Read the model definition and answer for the solid it produces. Units are mm, in the model's axes. Coordinates: 2 decimals unless noted, no trailing zeros. Write each loop counter-clockwise with the first axis right and the second up, starting at its lowest first coordinate (ties: lowest second). Pieces come first, ordered by that corner, then holes. Notation, with made-up numbers: (39, -9) -> (54, -9) arc R36 ccw to (54, 28) -> close; hole circle Ø4 at (-11, 56.5). An arc over 180 degrees is marked (long way). Use CSV: the item, a comma, the result in double quotes.
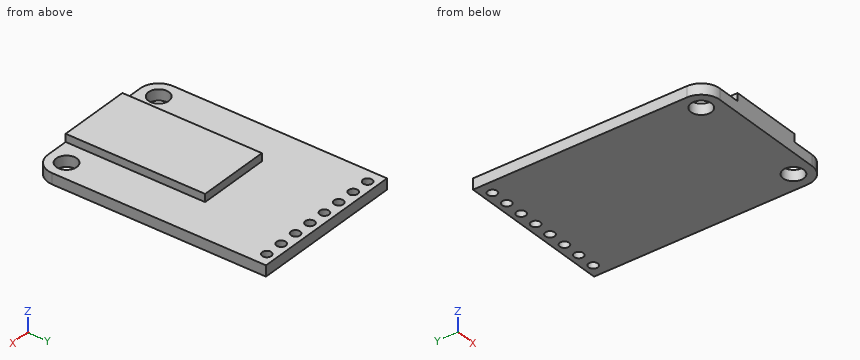
from build123d import *

# Parameters (mm, degrees)
F0_W     = 21.336
F0_H     = 31.75
F1_DEPTH = 1.4732
F2_R     = 2.54
F3_R     = 1.397
F4_DEPTH = 1.4732
F5_R     = 0.635
F6_DEPTH = 1.4732
F7_W     = 10.0076
F7_H     = 19.05
F8_DEPTH = 2.54


with BuildPart() as f1:
    # F0 (on Top) → F1 (new body)
    with BuildSketch(Plane.XY):
        Rectangle(F0_W, F0_H)
    extrude(amount=F1_DEPTH)

    # F2
    f2_edges = [f1.edges().sort_by_distance(p)[0] for p in [
        (10.668, -15.875, 0.7366),
        (-10.668, -15.875, 0.7366),
    ]]
    fillet(f2_edges, radius=F2_R)

    # F3 (on face) → F4 (cut, through all)
    with BuildSketch(Plane.XY.offset(1.4732)):
        with Locations((8.128, -13.335)):
            Circle(F3_R)
        with Locations((-8.128, -13.335)):
            Circle(F3_R)
    extrude(amount=-F4_DEPTH, mode=Mode.SUBTRACT)

    # F5 (on face) → F6 (cut, through all)
    with BuildSketch(Plane.XY.offset(1.4732)):
        with Locations((-8.89, 14.605)):
            Circle(F5_R)
        with Locations((-6.35, 14.605)):
            Circle(F5_R)
        with Locations((-3.81, 14.605)):
            Circle(F5_R)
        with Locations((-1.27, 14.605)):
            Circle(F5_R)
        with Locations((1.27, 14.605)):
            Circle(F5_R)
        with Locations((3.81, 14.605)):
            Circle(F5_R)
        with Locations((6.35, 14.605)):
            Circle(F5_R)
        with Locations((8.89, 14.605)):
            Circle(F5_R)
    extrude(amount=-F6_DEPTH, mode=Mode.SUBTRACT)

    # F7 (on face) → F8 (join)
    with BuildSketch(Plane(origin=(0, 0, 0), x_dir=(1, 0, 0), z_dir=(0, 0, -1))):
        with Locations((0, 6.35)):
            Rectangle(F7_W, F7_H)
    extrude(amount=-F8_DEPTH)


solid = f1.part
1. A cutting plane is placed at A-A (x = -6.35). Give the vertices of the cut face in (y, z) (3 decimals), and give its area (3 significant figures).
Solutions:
outline,"(-15.875, 0) -> (13.97, 0) -> (13.97, 1.473) -> (-15.875, 1.473) -> close; (15.24, 0) -> (15.875, 0) -> (15.875, 1.473) -> (15.24, 1.473) -> close"
area,"44.9 mm^2"
2. Each of these flat-tipped pins is pushed along its axis until it touches: pin 1 Ø0.9 at (y, z) = (-6, 2) entering from -X; pin 2 Ø1.7 at (x, y) = (-8.128, -13.335) entering from +Z; pin 3 Ø1.7 at (x, y) = (-1.27, 14.605) entering from +Z; pin 4 Ø0.9 at (y, z) = (-8, 2) entering from +X. Where does it stop, or does it pass through?
Solutions:
pin 1,"stops at x = -5"
pin 2,"passes through"
pin 3,"stops at z = 1.47"
pin 4,"stops at x = 5"
3. A cutting plane is placed at D-D (z = 0.4). Give the number of separate pieces and of enclosed holes in the cut face, and give its area (3 significant figures).
Solutions:
separate pieces,"1"
enclosed holes,"10"
area,"652 mm^2"
4. Find the intervals of material crossed by line 1 along Y through (x, z) = (-8, 0.8) (3 decimals); line 2 along Y through (x, z) = (9, 0.2) (3 decimals); line 3 along Y through (x, z) = (-3.81, 0.9) (3 decimals), in increasing order.
Solutions:
line 1,"y = -15.875 to -14.726, -11.944 to 15.875"
line 2,"y = -15.721 to -14.426, -12.244 to 13.98, 15.23 to 15.875"
line 3,"y = -15.875 to 13.97, 15.24 to 15.875"
5. A cutting plane is placed at C-C (x = -8.89). Give the vertices of the cut face in (y, z) (3 decimals), and give its area (3 significant figures).
Solutions:
outline,"(-15.758, 0) -> (-14.506, 0) -> (-14.506, 1.473) -> (-15.758, 1.473) -> close; (-12.164, 0) -> (13.97, 0) -> (13.97, 1.473) -> (-12.164, 1.473) -> close; (15.24, 0) -> (15.875, 0) -> (15.875, 1.473) -> (15.24, 1.473) -> close"
area,"41.3 mm^2"
6. A cutting plane is placed at B-B (y = -10). Give the vertices of the cut face in (x, z).
Solutions:
outline,"(-10.67, 0) -> (10.67, 0) -> (10.67, 1.47) -> (5, 1.47) -> (5, 2.54) -> (-5, 2.54) -> (-5, 1.47) -> (-10.67, 1.47) -> close"
